Autodesk Inventor part; units mm, degrees
ref_plane "YZ Plane" through (0, 0, 0) normal (1, 0, 0) x (0, 1, 0)
ref_plane "XZ Plane" through (0, 0, 0) normal (0, 1, 0) x (-1, 0, 0)
ref_plane "XY Plane" through (0, 0, 0) normal (0, 0, 1) x (1, 0, 0)
sketch "Sketch1" plane through (0, 0, 0) normal (0, 0, 1) x (1, 0, 0)
  line L0 (-28.2, -35.2) -> (28.2, -35.2)
  line L1 (35.2, -28.2) -> (35.2, 28.2)
  line L2 (28.2, 35.2) -> (-28.2, 35.2)
  line L3 (-35.2, 28.2) -> (-35.2, -28.2)
  line L4 (-35.2, -35.2) -> (35.2, 35.2) construction
  line L5 (35.2, -35.2) -> (-35.2, 35.2) construction
  arc A0 (-28.2, 35.2) -> (-35.2, 28.2) centre (-28.2, 28.2) ccw
  arc A1 (35.2, 28.2) -> (28.2, 35.2) centre (28.2, 28.2) ccw
  arc A2 (-35.2, -28.2) -> (-28.2, -35.2) centre (-28.2, -28.2) ccw
  arc A3 (28.2, -35.2) -> (35.2, -28.2) centre (28.2, -28.2) ccw
  line L6 (-2.5, -24.8747) -> (2.5, -24.8747) construction
  line L7 (2.5, 24.8747) -> (-2.5, 24.8747) construction
  line L8 (-2.5, -24.8747) -> (2.5, 24.8747) construction
  line L9 (2.5, -24.8747) -> (-2.5, 24.8747) construction
  arc A4 (-9.375, 23.1756) -> (-9.375, -23.1756) centre (0, 0) ccw
  arc A5 (9.375, -23.1756) -> (9.375, 23.1756) centre (0, 0) ccw
  arc A6 (-2.5, 18.5405) -> (-9.375, 23.1756) centre (-7.5, 18.5405) ccw
  arc A7 (9.375, 23.1756) -> (2.5, 18.5405) centre (7.5, 18.5405) ccw
  arc A8 (-9.375, -23.1756) -> (-2.5, -18.5405) centre (-7.5, -18.5405) ccw
  arc A9 (2.5, -18.5405) -> (9.375, -23.1756) centre (7.5, -18.5405) ccw
  line L10 (2.5, 4.3301) -> (2.5, 18.5405)
  line L11 (-2.5, 18.5405) -> (-2.5, 4.3301)
  line L12 (-2.5, -4.3301) -> (-2.5, -18.5405)
  line L13 (2.5, -18.5405) -> (2.5, -4.3301)
  arc A10 (-2.5, 4.3301) -> (-2.5, -4.3301) centre (0, 0) ccw
  arc A11 (2.5, -4.3301) -> (2.5, 4.3301) centre (0, 0) ccw
  dimension "d0" = 70.4
  dimension "d1" = 7
  dimension "d3" = 5
  dimension "d4" = 25
  dimension "d5" = 5
  dimension "d7" = 5
extrude "Extrusion1" add sketch "Sketch1" along normal blind 4.7
sketch "Sketch2" plane through (0, 0, 4.7) normal (0, 0, 1) x (1, 0, 0)
  circle A0 centre (0, 0) radius 27
  arc A1 (9.375, -23.1756) -> (9.375, 23.1756) centre (0, 0) ccw
  arc A2 (2.5, -18.5405) -> (9.375, -23.1756) centre (7.5, -18.5405) ccw
  line L0 (2.5, -18.5405) -> (2.5, -4.3301)
  arc A3 (2.5, -4.3301) -> (2.5, 4.3301) centre (0, 0) ccw
  line L1 (2.5, 4.3301) -> (2.5, 18.5405)
  arc A4 (9.375, 23.1756) -> (2.5, 18.5405) centre (7.5, 18.5405) ccw
  line L2 (-2.5, 18.5405) -> (-2.5, 4.3301)
  arc A5 (-2.5, 4.3301) -> (-2.5, -4.3301) centre (0, 0) ccw
  line L3 (-2.5, -4.3301) -> (-2.5, -18.5405)
  arc A6 (-9.375, -23.1756) -> (-2.5, -18.5405) centre (-7.5, -18.5405) ccw
  arc A7 (-9.375, 23.1756) -> (-9.375, -23.1756) centre (0, 0) ccw
  arc A8 (-2.5, 18.5405) -> (-9.375, 23.1756) centre (-7.5, 18.5405) ccw
  line L4 (28.2, 35.2) -> (-28.2, 35.2)
  arc A9 (-28.2, 35.2) -> (-35.2, 28.2) centre (-28.2, 28.2) ccw
  line L5 (-35.2, 28.2) -> (-35.2, -28.2)
  arc A10 (-35.2, -28.2) -> (-28.2, -35.2) centre (-28.2, -28.2) ccw
  line L6 (-28.2, -35.2) -> (28.2, -35.2)
  arc A11 (28.2, -35.2) -> (35.2, -28.2) centre (28.2, -28.2) ccw
  line L7 (35.2, -28.2) -> (35.2, 28.2)
  arc A12 (35.2, 28.2) -> (28.2, 35.2) centre (28.2, 28.2) ccw
  dimension "d10" = 54
extrude "Extrusion2" add sketch "Sketch2" along normal blind 2 contours A0
sketch "Sketch3" plane through (0, 0, 0) normal (0, 0, -1) x (-1, 0, 0)
  line L0 (-27.5, -27.5) -> (27.5, -27.5) construction
  line L1 (27.5, -27.5) -> (27.5, 27.5) construction
  line L2 (27.5, 27.5) -> (-27.5, 27.5) construction
  line L3 (-27.5, 27.5) -> (-27.5, -27.5) construction
  line L4 (-27.5, -27.5) -> (27.5, 27.5) construction
  line L5 (27.5, -27.5) -> (-27.5, 27.5) construction
  line L6 (27.5, 27.5) -> (32.8233, 32.8233) construction
  line L7 (29.2678, 25.7322) -> (34.5911, 31.0555)
  line L8 (31.0555, 34.5911) -> (25.7322, 29.2678)
  arc A0 (25.7322, 29.2678) -> (29.2678, 25.7322) centre (27.5, 27.5) ccw
  arc A1 (34.5911, 31.0555) -> (31.0555, 34.5911) centre (32.8233, 32.8233) ccw
  arc A2 (35.2, 28.2) -> (28.2, 35.2) centre (28.2, 28.2) ccw construction
  line L9 (-25.7322, 29.2678) -> (-31.0555, 34.5911)
  arc A3 (-29.2678, 25.7322) -> (-25.7322, 29.2678) centre (-27.5, 27.5) ccw
  line L10 (-34.5911, 31.0555) -> (-29.2678, 25.7322)
  arc A4 (-31.0555, 34.5911) -> (-34.5911, 31.0555) centre (-32.8233, 32.8233) ccw
  line L11 (-29.2678, -25.7322) -> (-34.5911, -31.0555)
  arc A5 (-25.7322, -29.2678) -> (-29.2678, -25.7322) centre (-27.5, -27.5) ccw
  line L12 (-31.0555, -34.5911) -> (-25.7322, -29.2678)
  arc A6 (-34.5911, -31.0555) -> (-31.0555, -34.5911) centre (-32.8233, -32.8233) ccw
  line L13 (25.7322, -29.2678) -> (31.0555, -34.5911)
  arc A7 (29.2678, -25.7322) -> (25.7322, -29.2678) centre (27.5, -27.5) ccw
  line L14 (34.5911, -31.0555) -> (29.2678, -25.7322)
  arc A8 (31.0555, -34.5911) -> (34.5911, -31.0555) centre (32.8233, -32.8233) ccw
  point P0 (0, 0)
  point P1 (30.1617, 30.1617)
  dimension "d13" = 55
  dimension "d14" = 5
  dimension "d18" = 360
extrude "Extrusion3" cut sketch "Sketch3" against normal through all
chamfer "Chamfer1" distance 2.5 angle 45 12 edges at (28.3939, 31.9294, 0) (25.7322, 25.7322, 0) (31.9294, 28.3939, 0) (-28.3939, 31.9294, 0) (-25.7322, 25.7322, 0) (-31.9294, 28.3939, 0) (-25.7322, -25.7322, 0) (-31.9294, -28.3939, 0) (-28.3939, -31.9294, 0) (25.7322, -25.7322, 0) (28.3939, -31.9294, 0) (31.9294, -28.3939, 0)
fillet "Fillet1" radius 1 8 edges at (31.0555, 34.5911, 3.6) (34.5911, 31.0555, 3.6) (34.5911, -31.0555, 3.6) (31.0555, -34.5911, 3.6) (-31.0555, -34.5911, 3.6) (-34.5911, -31.0555, 3.6) (-34.5911, 31.0555, 3.6) (-31.0555, 34.5911, 3.6)
hole "Hole1" at (0, 0, 0) direction (0, 0, 1) diameter 4.2 end through all
sketch "Sketch4" plane through (0, 0, 0) normal (0, 0, -1) x (-1, 0, 0)
  line L0 (-35.2, 35.2) -> (-2.5, 35.2)
  line L1 (-2.5, 35.2) -> (-2.5, 4.3301)
  line L2 (-2.5, 4.3301) -> (-4.2, 4.3301)
  line L3 (-4.2, 4.3301) -> (-4.2, -19.8)
  line L4 (-4.2, -19.8) -> (-35.2, -19.8)
  line L5 (-35.2, 28.1289) -> (-35.2, -28.1289) construction
  line L6 (-35.2, 35.2) -> (-35.2, -19.8)
  line L7 (-2.5, 18.5405) -> (-2.5, 4.3301)
  line L8 (28.1289, 35.2) -> (-28.1289, 35.2) construction
  point P0 (0, 0)
  point P1 (2.5, 4.3301)
  dimension "d39" = 31
  dimension "d41" = 55
extrude "Extrusion4" cut sketch "Sketch4" against normal through all
fillet "Fillet2" radius 1 2 edges at (35.2, -19.8, 2.35) (15.263, -19.8, 3.35)
equation "\"Offset\" = 0.3"
properties part number "V4 In wall"
Geometry: final body of the model. Coordinates: model frame, mm. A direction names the side the tool comes from. Round coordinates to 2 decimals unless told otherwise and drop trailing zeros. Loops run counter-clockwise (first coordinate to the right, second up) from the corner with the lowest first, then second, coordinate; pieces in that order, holes last. Notation, with made-up numbers: M -25.5,54 L -15.5,54 A15 ccw -15.5,79 Z; hole C 37.5,68 d4. An arc over 180 degrees is marked long. Put each result on its own line as item: value. Start each with the question number.
(1) Section query A-A (y = -1). Return loops of the section in (x, z), then the cut area to 3 significant figures.
(2) Contact query for flat-ended pins moving along their axis: pin 1 Ø3.5 at (y, z) = (18, 3) entering from +X; pin 2 Ø1.6 at (y, z) = (0, 2.5) entering from +X; pin 3 Ø2.5 at (x, y) = (0, 0) entering from +Z; pin 4 Ø3.5 at (x, z) = (22.5, 2) entering from +Y. Output: stop coordinate, or through.
(3) Set-up query: faces 4 (the face through (-13, 35.2, 2)), 5 (the face through (-2.5, -11, 3)), 6 (the face through (2.5, -12, 3)). Return all of +Z, -Z, +X, -X, +Y, -Y with unobstructed straight access to the full face (end or side cutting, diameter ignored); none if empty.
(4) Draft query along Y for faces 1 (the face through (-21, -18, 4.7)), 2 (the face through (0, -35.2, 2)), 3 (the face through (-5, 0, 3)). Return one class per face: +Y half, -Y half, draft (parallel to the pull), parting line (faces both ways), or undercut.
(5) Material intervals for line 1 along X through (y, z) = (-0.5, 5.5); line 2 along Y through (x, z) = (0, 4.25); line 3 along Y through (x, z) = (-4, 3), sorted ascending. Write a range as [from, to].
Findings below:
1. outline: M -35.2,0 L -24.98,0 L -24.98,6.7 L -26.98,6.7 L -26.98,4.7 L -35.2,4.7 Z; M -4.9,0 L -1.85,0 L -1.85,6.7 L -4.9,6.7 Z; M 1.85,0 L 4.2,0 L 4.2,6.7 L 1.85,6.7 Z
1. area: 88.3 mm2
2. pin 1: stops at x = 2.5
2. pin 2: stops at x = 4.2
2. pin 3: passes through
2. pin 4: stops at y = -19.8
3. face 4: +Z, -Z, +X, -X, +Y
3. face 5: +Z, -Z
3. face 6: +Z, -Z, +X
4. face 1: draft
4. face 2: -Y half
4. face 3: undercut
5. line 1: x = [-27, -24.99], [-4.97, -2.04], [2.04, 4.2]
5. line 2: y = [-35.2, -2.1], [2.1, 35.2]
5. line 3: y = [-35.2, -22.11], [-3, 3], [22.11, 35.2]
